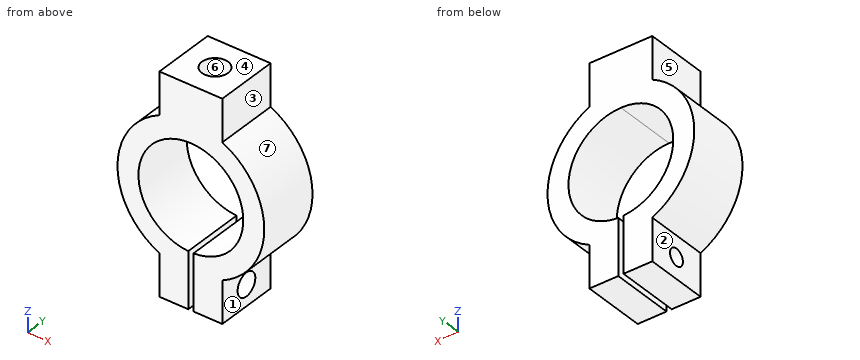
```python
from build123d import *

# Parameters (mm, degrees)
LOOP_SKETCH_R                   = 7
LOOP_SKETCH_R_2                 = 5
LOOP_EXTRUDE_DEPTH              = 6
BLOCK_SKETCH_W                  = 6
BLOCK_SKETCH_H                  = 4
BLOCK_EXTRUDE_DEPTH             = 6
SLOT_SKETCH_W                   = 0.5
SLOT_SKETCH_H                   = 5.330809231
SLOT_CUT_DEPTH                  = 6
M3X0_5_TAPPED_HOLE1_D           = 2.5
M3X0_5_TAPPED_HOLE1_DEPTH       = 4
M3X0_5_TAPPED_HOLE1_TIP         = 0.751075774
F_2_2_2_2_DIAMETER_HOLE1_REACH  = 17.576
F_2_2_2_2_DIAMETER_HOLE1_BORE_R = 1.1
M2X0_4_TAPPED_HOLE1_D           = 1.6


with BuildPart() as part:
    # Loop Sketch → Loop Extrude (new body)
    with BuildSketch(Plane(origin=(0, 0, 0), x_dir=(1, 0, 0), z_dir=(0, 1, 0))):
        with Locations(Location((0, 0, 0), (0, 0, 270))):
            Circle(LOOP_SKETCH_R)
        with Locations(Location((0, 0, 0), (0, 0, 270))):
            Circle(LOOP_SKETCH_R_2, mode=Mode.SUBTRACT)
    extrude(amount=LOOP_EXTRUDE_DEPTH)

    # Block Sketch → Block Extrude (add)
    with BuildSketch(Plane(origin=(0, 0, 0), x_dir=(1, 0, 0), z_dir=(0, 1, 0))):
        with Locations((0, -8.32455532)):
            Rectangle(BLOCK_SKETCH_W, BLOCK_SKETCH_H)
        with Locations((0, 8.32455532)):
            Rectangle(BLOCK_SKETCH_W, BLOCK_SKETCH_H)
    extrude(amount=BLOCK_EXTRUDE_DEPTH)

    # Slot Sketch → Slot Cut (cut)
    with BuildSketch(Plane(origin=(0, 0, 0), x_dir=(1, 0, 0), z_dir=(0, 1, 0))):
        with Locations((0, 7.659150705)):
            Rectangle(SLOT_SKETCH_W, SLOT_SKETCH_H)
    extrude(amount=SLOT_CUT_DEPTH, mode=Mode.SUBTRACT)

    # M3x0.5 Tapped Hole1
    with Locations(Plane.XY.offset(10.32455532)):
        with Locations((0, 3)):
            Hole(M3X0_5_TAPPED_HOLE1_D / 2, depth=M3X0_5_TAPPED_HOLE1_DEPTH)
            with Locations((0, 0, -(M3X0_5_TAPPED_HOLE1_DEPTH + M3X0_5_TAPPED_HOLE1_TIP / 2))):  # 118° drill point
                Cone(0, M3X0_5_TAPPED_HOLE1_D / 2, M3X0_5_TAPPED_HOLE1_TIP, mode=Mode.SUBTRACT)

    # Ø2.2 (2.2) Diameter Hole1 bore → Ø2.2 (2.2) Diameter Hole1 (cut, up to next)
    with BuildSketch(Plane(origin=(3, 0, 0), x_dir=(0, 0, -1), z_dir=(1, 0, 0)), mode=Mode.PRIVATE) as f_2_2_2_2_diameter_hole1_sk1:
        with Locations((8.32455532, 3)):
            Circle(F_2_2_2_2_DIAMETER_HOLE1_BORE_R)
    f_2_2_2_2_diameter_hole1_tool1 = extrude(f_2_2_2_2_diameter_hole1_sk1.sketch, amount=-F_2_2_2_2_DIAMETER_HOLE1_REACH, mode=Mode.PRIVATE) & part.part
    add(f_2_2_2_2_diameter_hole1_tool1.solids().sort_by_distance((3, 3, -8.324555))[0], mode=Mode.SUBTRACT)

    # M2x0.4 Tapped Hole1 (through all)
    with Locations(Plane(origin=(-0.25, 0, 0), x_dir=(0, 0, -1), z_dir=(1, 0, 0))):
        with Locations((8.32455532, 3)):
            Hole(M2X0_4_TAPPED_HOLE1_D / 2)


solid = part.part
```
CAD build for the part. Positions are in the model's coordinates, mm. Face numbers are marked on the shaded views. A direction names the side the tool comes from. Round coordinates to 2 decimals unless told otherwise and drop trailing zeros. Order: outer loops, then holes, each group sorted by start corner. A loop starts at its lowest first (then second) coordinate and runs counter-clockwise, first axis right, second up.
Item 1: Tool access for the marked faces 1, 2, 3 and 4: list every direction of +Z, -Z, +X, -X, +Y, -Y with a clear straight run to the whole face (end or side of a thin tool).
Item 2: Saw through at B-B on y = 0.5. Write the cut outline in (x, z).
Item 3: Mould opens along X. For the marked faces 5, 6 and 7 say: pulls with the +X half, pulls with the -X half, needs draft (parallel to the pull), parting line crosses it, or undercut.
Item 4: Saw through at D-D on x = -4.75. Write the cut outline in (y, z).
Item 5: Probe line 1 along X through (y, z) = (3, 8.6); line 2 along Z through (x, y) = (2.75, 2.3); line 3 along Y through (x, z) = (0, 7.4). List the from-to ranges inside material, lowest first.
Item 6: Saw through at A-A on z = 0. Write the cut outline in (x, y).
Item 7: Pin check, flat tips, straight feed: pin 1 (2 mm diameter, centred on y = 3, z = -8.32, fed in from +X); pin 2 (1 mm diameter, centred on x = 5, y = 2, fed in from -Z); pin 3 (1 mm diameter, centred on y = 1.5, z = 5, fed in from -X). Stop position of each tip, or through.
Item 8: Saw through at C-C on x = 2.75. Write the cut outline in (y, z).
Reported:
1. face 1: -Z, +X, +Y, -Y
1. face 2: -Z, -X, +Y, -Y
1. face 3: +Z, +X, +Y, -Y
1. face 4: +Z, +X, -X, +Y, -Y
2. outline: (-3, -10.32) - (-0.25, -10.32) - (-0.25, -4.99) arc R5 cw (long way) to (0.25, -4.99) - (0.25, -10.32) - (3, -10.32) - (3, -6.32) arc R7 ccw to (3, 6.32) - (3, 10.32) - (-3, 10.32) - (-3, 6.32) arc R7 ccw to (-3, -6.32) - close
3. face 5: pulls with the -X half
3. face 6: undercut
3. face 7: pulls with the +X half
4. outline: (0, -5.14) - (6, -5.14) - (6, -1.56) - (0, -1.56) - close; (0, 1.56) - (6, 1.56) - (6, 5.14) - (0, 5.14) - close
5. line 1: x = -3 to -1.25, 1.25 to 3
5. line 2: z = -10.32 to -9.17, -7.48 to -4.18, 4.18 to 10.32
5. line 3: y = 0 to 1.75, 4.25 to 6
6. outline: (-7, 0) - (-5, 0) - (-5, 6) - (-7, 6) - close; (5, 0) - (7, 0) - (7, 6) - (5, 6) - close
7. pin 1: stops at x = -0.25
7. pin 2: stops at z = -5.36
7. pin 3: stops at x = -5.36
8. outline: (0, -10.32) - (6, -10.32) - (6, -4.18) - (0, -4.18) - close; (0, 4.18) - (6, 4.18) - (6, 10.32) - (0, 10.32) - close; hole circle Ø2.2 at (3, -8.32)
